Source: CAD feature listing. Evaluate the final solid. Frame: model axes, mm. A direction names the side the tool comes from. Give positions to 0.01 mm unless a question says otherwise; leave off trailing zeros. Write each loop counter-clockwise with the first axis right and the second up, starting at its lowest first coordinate (ties: lowest second). Pieces come first, ordered by that corner, then holes. Notation, with made-up numbers: (20.25, 17.5) - (26.25, 17.5) arc R8 cw to (26.25, 29.5) - close; hole circle Ø5 at (-33.5, 23). An arc over 180 degrees is marked (long way). Answer as a JSON object with one key per item and string values. Group by question number.
from build123d import *

# Parameters (mm, degrees)
SKETCH_1_W                  = 30
SKETCH_1_H                  = 30
EXTRUDE_1_DEPTH             = 2
SKETCH_2_R                  = 4
EXTRUDE_2_DEPTH             = 9.5
SKETCH_3_R                  = 4
EXTRUDE_3_DEPTH             = 9.5
CUT_EXTRUDE_START           = -30
SKETCH_4_R                  = 3.5
CUT_EXTRUDE_1_DEPTH         = 30
EXTRUDE_4_DEPTH             = 9.5
EXTRUDE_START               = -9.5
EXTRUDE_5_DEPTH             = 9.5
HOLE_WIZARD_M41_D           = 4.5
HOLE_WIZARD_M41_DEPTH       = 21
HOLE_WIZARD_M41_CSINK_D     = 9.4
HOLE_WIZARD_M41_CSINK_ANGLE = 90
HOLE_WIZARD_M41_TIP         = 1.351936393


with BuildPart() as part:
    # Sketch 1 → Extrude 1 (new body)
    with BuildSketch(Plane(origin=(0, 0, 0), x_dir=(1, 0, 0), z_dir=(0, 1, 0))):
        with Locations((-70.332590066, -54.606104746)):
            Rectangle(SKETCH_1_W, SKETCH_1_H)
    extrude(amount=EXTRUDE_1_DEPTH)



with BuildPart() as body_2:
    # Sketch 2 → Extrude 2 (new body)
    with BuildSketch(Plane.ZY.offset(85.332590066)):
        with Locations((37.577272985, 5.447294836)):
            Circle(SKETCH_2_R)
    extrude(amount=-EXTRUDE_2_DEPTH)


with BuildPart() as body_3:
    # Sketch 3 → Extrude 3 (new body)
    with BuildSketch(Plane.ZY.offset(64.832590066)):
        with Locations((37.577272985, 5.447294836)):
            Circle(SKETCH_3_R)
    extrude(amount=-EXTRUDE_3_DEPTH)


with BuildPart() as cut_extrude_1_tool:
    # Sketch 4 → Cut-Extrude 1 (new body)
    with BuildSketch(Plane.ZY.offset(85.332590066).offset(CUT_EXTRUDE_START)):
        with Locations((37.577272985, 5.447294836)):
            Circle(SKETCH_4_R)
    extrude(amount=CUT_EXTRUDE_1_DEPTH)


with BuildPart() as body_2_1:
    add(body_2.part)

    # Cut-Extrude 1: cut by cut_extrude_1_tool
    add(cut_extrude_1_tool.part, mode=Mode.SUBTRACT)


with BuildPart() as body_3_1:
    add(body_3.part)

    # Cut-Extrude 1: cut by cut_extrude_1_tool
    add(cut_extrude_1_tool.part, mode=Mode.SUBTRACT)


with BuildPart() as part_1:
    add(part.part)

    add(body_2_1.part)  # Extrude 4 merges body 2
    # Sketch 5 → Extrude 4 (add)
    with BuildSketch(Plane.ZY.offset(85.332590066)):
        with BuildLine():
            Line((39.606104746, 0), (36.267042135, 1.667970145))
            ThreePointArc((36.267042135, 1.667970145), (39.413946145, 1.89389763), (41.418204347, 4.330493028))
            Line((41.418204347, 4.330493028), (41.418204347, 0))
            Line((41.418204347, 0), (39.606104746, 0))
        make_face()
    extrude(amount=-EXTRUDE_4_DEPTH)


    add(body_3_1.part)  # Extrude 5 merges body 3
    # Sketch 6 → Extrude 5 (add)
    with BuildSketch(Plane.ZY.offset(64.832590066).offset(EXTRUDE_START)):
        with BuildLine():
            Line((41.418204347, 2), (41.418204347, 4.330493028))
            Line((41.418204347, 4.330493028), (40.83906741, 4.178162405))
            ThreePointArc((40.83906741, 4.178162405), (39.143105824, 2.317092363), (36.636762804, 2.076027923))
            Line((36.636762804, 2.076027923), (36.267042135, 1.667970145))
            Line((36.267042135, 1.667970145), (39.606104746, 0))
            Line((39.606104746, 0), (41.418204347, 2))
        make_face()
    extrude(amount=EXTRUDE_5_DEPTH)

    # Hole Wizard M41
    with Locations(Plane(origin=(0, 2, 0), x_dir=(1, 0, 0), z_dir=(0, 1, 0))):
        with Locations((-62.832590066, -48.465179446), (-77.832590066, -62.559129646)):
            CounterSinkHole(HOLE_WIZARD_M41_D / 2, HOLE_WIZARD_M41_CSINK_D / 2, depth=HOLE_WIZARD_M41_DEPTH, counter_sink_angle=HOLE_WIZARD_M41_CSINK_ANGLE)
            with Locations((0, 0, -(HOLE_WIZARD_M41_DEPTH + HOLE_WIZARD_M41_TIP / 2))):  # 118° drill point
                Cone(0, HOLE_WIZARD_M41_D / 2, HOLE_WIZARD_M41_TIP, mode=Mode.SUBTRACT)


solid = part_1.part
Q1. Section A-A on y = 7. Return the cut outline in (x, z), then the cut area to 3 significant figures.
Q2. Section D-D on x = -63. State how many separate pieces and enclosed holes the cut face has, then the cut area to 3 significant figures.
Q3. Section B-B on y = 1. Return the cut outline in (x, z), then the cut area to 3 significant figures.
Q4. Reachability of faces 5 (the flat face through (-71, 0, 54)), 6 (the flat face through (-81, 3, 41.418)), 7 (the flat face through (-70, 1, 39.606)), 8 (the flat face through (-75.833, 2.6, 40)) from +Z, -Z, +X, -X, +Y, -Y: full face, straight path, thin tool, end or side. Return the list, or none.
Q5. First-contact query: pin 1 Ø2 at (x, z) = (-82, 49) entering from +Y; pin 2 Ø1.6 at (x, y) = (-70, 1) entering from -Z; pin 3 Ø0.7 at (x, y) = (-60.5, 3) entering from +Z. Flat tips, straight axial feed; report the tip coordinate or a pass-through.
Q6. Section C-C on z = 38.5. Return the cut outline in (x, y), then the cut area to 3 significant figures.
Q7. Draft query along Z for faces 1 (the cylindrical face through (-60.15, 9.06, 35.86)), 2 (the flat face through (-60.016, 0.846, 37.913)), 3 (the cylindrical face through (-80.52, 4.11, 40.81)), 4 (the flat face through (-71, 2, 54)). Return one class per face: released by +Z, released by -Z, zero draft, split by the parting line, or undercut.
Q8. Ray query, probe 1 along X at (y, z) = (1, 45.5); probe 2 along Y at (x, z) = (-58.75, 39.5); probe 3 along Y at (x, z) = (-72, 57.5). Return the intervals inside material, ascending. Write a range as [from, to].
Taken from the geometry:
{
 "1": {"outline": "(-85.33, 33.89) - (-75.83, 33.89) - (-75.83, 34.44) - (-85.33, 34.44) - close; (-85.33, 40.71) - (-75.83, 40.71) - (-75.83, 41.26) - (-85.33, 41.26) - close; (-64.83, 33.89) - (-55.33, 33.89) - (-55.33, 34.44) - (-64.83, 34.44) - close; (-64.83, 40.71) - (-55.33, 40.71) - (-55.33, 41.26) - (-64.83, 41.26) - close", "area": "20.9 mm²"},
 "2": {"separate pieces": "2", "enclosed holes": "1", "area": "61.1 mm²"},
 "3": {"outline": "(-85.33, 37.6) - (-75.83, 37.6) - (-75.83, 39.61) - (-64.83, 39.61) - (-64.83, 37.6) - (-55.33, 37.6) - (-55.33, 69.61) - (-85.33, 69.61) - close; hole circle Ø7.4 at (-77.83, 62.56); hole circle Ø7.4 at (-62.83, 48.47)", "area": "852 mm²"},
 "4": {"face 5": "+Z, -Z, +X, -X, -Y", "face 6": "+Z, +X, -X", "face 7": "-Z, +Y, -Y", "face 8": "-Z, +Y"},
 "5": {"pin 1": "stops at y = 2", "pin 2": "stops at z = 39.61", "pin 3": "stops at z = 41.42"},
 "6": {"outline": "(-85.33, 0.55) - (-75.83, 0.55) - (-75.83, 2.07) - (-85.33, 2.07) - close; (-85.33, 8.82) - (-75.83, 8.82) - (-75.83, 9.34) - (-85.33, 9.34) - close; (-64.83, 0.55) - (-55.33, 0.55) - (-55.33, 2.07) - (-64.83, 2.07) - close; (-64.83, 8.82) - (-55.33, 8.82) - (-55.33, 9.34) - (-64.83, 9.34) - close", "area": "38.7 mm²"},
 "7": {"face 1": "split by the parting line", "face 2": "released by -Z", "face 3": "undercut", "face 4": "zero draft"},
 "8": {"probe 1": "x = [-85.33, -65.05], [-60.62, -55.33]", "probe 2": "y = [0.05, 2.52], [8.37, 8.95]", "probe 3": "y = [0, 2]"}
}
